Check sheet for the modelled part. Datum: model origin and axes. Units: mm. A direction names the side the tool comes from. Round coordinates to 2 decimals unless told otherwise and drop trailing zeros. Loops run counter-clockwise (first coordinate to the right, second up) from the corner with the lowest first, then second, coordinate; pieces in that order, holes last. Notation, with made-up numbers: (-17.75, 81) -> (26.25, 81) arc R3 cw to (26.25, 86) -> close; hole circle Ø10 at (41, 48.5). An arc over 180 degrees is marked (long way). Return JSON: item names as keys, results as strings.
from build123d import *

# Parameters (mm, degrees)
SKETCH1_R                = 60
BOSS_EXTRUDE1_DEPTH      = 200
BOSS_EXTRUDE1_DEPTH_BACK = 50
SKETCH2_R                = 75
SKETCH2_R_2              = 12.5
CUT_EXTRUDE1_DEPTH       = 50
FILLET1_R                = 10


with BuildPart() as part:
    # Sketch1 → Boss-Extrude1 (new body, two sides)
    with BuildSketch(Plane(origin=(0, 0, 0), x_dir=(0, 0, -1), z_dir=(1, 0, 0))) as boss_extrude1_sk:
        Circle(SKETCH1_R)
    extrude(amount=BOSS_EXTRUDE1_DEPTH)
    extrude(boss_extrude1_sk.sketch, amount=-BOSS_EXTRUDE1_DEPTH_BACK)

    # Sketch2 → Cut-Extrude1 (cut)
    with BuildSketch(Plane.ZY.offset(50)):
        Circle(SKETCH2_R)
        Circle(SKETCH2_R_2, mode=Mode.SUBTRACT)
    extrude(amount=-CUT_EXTRUDE1_DEPTH, mode=Mode.SUBTRACT)

    # Fillet1
    fillet1_edges = [part.edges().sort_by_distance(p)[0] for p in [
        (0, 0, 60),
        (200, 0, 60),
    ]]
    fillet(fillet1_edges, radius=FILLET1_R)


solid = part.part
Q1. Section check A-A (y = 0). Record the boundary of the cut face in (x, z), then the cut area to 3 significant figures.
Results list:
{"outline": "(-50, -12.5) -> (0, -12.5) -> (0, -50) arc R10 ccw to (10, -60) -> (190, -60) arc R10 ccw to (200, -50) -> (200, 50) arc R10 ccw to (190, 60) -> (10, 60) arc R10 ccw to (0, 50) -> (0, 12.5) -> (-50, 12.5) -> close", "area": "25,200 mm^2"}
Q2. Material ranges on line 1 (X direction, y = -34, z = 7); line 2 (Z direction, x = 188, y = 2); line 3 (Y direction, x = 157, z = -16), recorded low to high.
Results list:
{"line 1": "0 to 200", "line 2": "-59.97 to 59.97", "line 3": "-57.83 to 57.83"}
Q3. Tool access check on faces 1 (the cylindrical face through (-25.35, 3.755, 11.923)), 2 (the flat face through (200, 1, 1)). Record the directions out of +Z, -Z, +X, -X, +Y, -Y that give a thin tool (end or side, any length) a straight path to the whole face; none if there is none.
Results list:
{"face 1": "-X", "face 2": "+Z, -Z, +X, +Y, -Y"}
Q4. Section check C-C (x = 123). Record the boundary of the cut face in (y, z).
Results list:
{"outline": "circle Ø120 at (0, 0)"}
Q5. Go/stop test with flat-tipped pins: pin 1 (12 mm diameter, centred on x = 63, y = 30, fed in from -Z); pin 2 (10 mm diameter, centred on y = -15, z = 19, fed in from -X); pin 3 (5 mm diameter, centred on x = 38.5, y = 44.5, fed in from -Z). Record where each tip stops, or that it passes through.
Results list:
{"pin 1": "z = -54.99", "pin 2": "x = 0", "pin 3": "z = -42.85"}
